Autodesk Inventor part; units mm, degrees
ref_plane "YZ Plane" through (0, 0, 0) normal (1, 0, 0) x (0, 1, 0)
ref_plane "XZ Plane" through (0, 0, 0) normal (0, 1, 0) x (-1, 0, 0)
ref_plane "XY Plane" through (0, 0, 0) normal (0, 0, 1) x (1, 0, 0)
sketch "Sketch1" plane through (0, 0, 0) normal (0, 1, 0) x (-1, 0, 0)
  line L0 (24, -38) -> (28.2, -38)
  line L1 (28.2, -38) -> (28.2, -55.6)
  line L2 (28.2, -55.6) -> (24, -55.6)
  line L3 (24, -55.6) -> (24, -38)
  line L4 (24, -38) -> (27, -38)
  line L5 (27, -38) -> (27, -42)
  line L6 (27, -42) -> (24, -42)
  line L7 (24, -42) -> (24, -38)
  line L8 (27, -42) -> (28.2, -42)
  line L9 (28.2, -42) -> (28.2, -38)
  line L10 (28.2, -38) -> (27, -38)
  line L11 (27, -38) -> (27, -42)
  point P0 (0, 0)
  dimension "d0" = 4.2
  dimension "d1" = 17.6
  dimension "d2" = 3
  dimension "d3" = 4
revolve "Revolution1" add sketch "Sketch1" angle 360 about axis through (-24, 0, -55.6) along (0, 0, 1) contours L0 L5 L6 L3 | L6 L8 L1 L2 L3
sketch "Sketch2" plane through (-24, 0, -42) normal (0, 0, 1) x (1, 0, 0)
  circle A0 centre (0, 0) radius 3
  circle A1 centre (0, 0) radius 4.2
  line L0 (0, 4.2) -> (3.6373, 2.1)
  line L1 (3.6373, 2.1) -> (3.6373, -2.1)
  line L2 (3.6373, -2.1) -> (0, -4.2)
  line L3 (0, -4.2) -> (-3.6373, -2.1)
  line L4 (-3.6373, -2.1) -> (-3.6373, 2.1)
  line L5 (-3.6373, 2.1) -> (0, 4.2)
  point P0 (24, 0)
  point P1 (-3.6373, 2.1)
  point P2 (-3.6373, 2.1)
  point P3 (-3.6373, -2.1)
  point P4 (-3.6373, -2.1)
  point P5 (0, -4.2)
  point P6 (0, -4.2)
  point P7 (3.6373, 2.1)
  point P8 (3.6373, 2.1)
extrude "Extrusion1" cut sketch "Sketch2" against normal blind 3 contours A1 L1 | L0 A1 | A1 L2 | L5 A1 | A1 L3 | L4 A1
properties part number "pm6m6 fitting dtraight"
Part model, mm, in its own coordinate system. A direction names the side the tool comes from. Coordinates: 2 decimals unless noted, no trailing zeros. Write each loop counter-clockwise with the first axis right and the second up, starting at its lowest first coordinate (ties: lowest second). Pieces come first, ordered by that corner, then holes.
Item 1: Slice it at C-C (x = -24.5). Write the cut outline in (y, z).
Item 2: Which spindle directions (+Z, -Z, +X, -X, +Y, -Y) get a long thin tool onto all of the face, cutting with end or side? Do faces 1 (the face through (-22.207, 3.165, -43.479)), 2 (the face through (-22.156, -3.135, -43.479)), 3 (the face through (-26, -3.4, -45)). Say none if no direction does.
Item 3: Slice it at B-B (z = -43.75). Write the cut outline in (x, y).
Item 4: Probe line 1 (X direction, y = 1, z = -44.5); line 2 (Z direction, x = -25.75, y = -3.5); line 3 (Z direction, x = -27, y = 1.5). List the from-to ranges inside material, lowest first.
Item 5: Slice it at A-A (y = 0). Write the cut outline in (x, z), and give its area (3 significant figures).
Item 6: Pin check, flat tips, straight feed: pin 1 (1.5 mm diameter, centred on x = -23.5, z = -48.5, fed in from +Y); pin 2 (1.5 mm diameter, centred on y = -1.5, z = -51.5, fed in from -X); pin 3 (0.9 mm diameter, centred on y = 1, z = -44, fed in from -X); pin 4 (4 mm diameter, centred on x = -21, z = -52, fed in from +Y). Stop position of each tip, or through.
Item 7: Slice it at D-D (y = -3.25). Write the cut outline in (x, z), and give its area (3 significant figures).
Results found:
1. outline: (-4.17, -55.6) - (4.17, -55.6) - (4.17, -45) - (3.91, -45) - (3.91, -42) - (2.96, -42) - (2.96, -38) - (-2.96, -38) - (-2.96, -42) - (-3.91, -42) - (-3.91, -45) - (-4.17, -45) - close
2. face 1: +Z, +X, +Y
2. face 2: +Z, +X, -Y
2. face 3: +Z, -X, -Y
3. outline: (-27.64, -2.1) - (-24, -4.2) - (-20.36, -2.1) - (-20.36, 2.1) - (-24, 4.2) - (-27.64, 2.1) - close
4. line 1: x = -27.64 to -20.36
4. line 2: z = -55.6 to -45
4. line 3: z = -55.6 to -42
5. outline: (-28.2, -55.6) - (-19.8, -55.6) - (-19.8, -45) - (-20.36, -45) - (-20.36, -42) - (-21, -42) - (-21, -38) - (-27, -38) - (-27, -42) - (-27.64, -42) - (-27.64, -45) - (-28.2, -45) - close
5. area: 135 mm2
6. pin 1: stops at y = 4.2
6. pin 2: stops at x = -28.13
6. pin 3: stops at x = -27.64
6. pin 4: stops at y = 4.08
7. outline: (-26.66, -55.6) - (-21.34, -55.6) - (-21.34, -45) - (-22.35, -45) - (-22.35, -42) - (-25.65, -42) - (-25.65, -45) - (-26.66, -45) - close
7. area: 66.3 mm2
